```python
from build123d import *

# Parameters (mm, degrees)
BOSS_EXTRUDE1_DEPTH = 25.4
CUT_EXTRUDE1_DEPTH  = 9.5
SKETCH5_W           = 25.4
SKETCH5_H           = 42.164
BOSS_EXTRUDE2_DEPTH = 11.43
CUT_EXTRUDE2_REACH  = 53.538
CUT_EXTRUDE3_REACH  = 53.255
CUT_EXTRUDE4_DEPTH  = 20
SKETCH10_W          = 19.05
SKETCH10_H          = 19.05
CUT_EXTRUDE5_DEPTH  = 26.289
CUT_EXTRUDE6_REACH  = 55.322
SKETCH11_W          = 1.5875
SKETCH11_H          = 12.7
SKETCH12_R          = 0.9921875
CUT_EXTRUDE7_DEPTH  = 51.724378715
CUT_EXTRUDE8_REACH  = 52.836
SKETCH13_R          = 0.9921875
CUT_EXTRUDE9_START  = -7.875
CUT_EXTRUDE9_DEPTH  = 1.225
CUT_EXTRUDE10_START = 7.875
CUT_EXTRUDE10_DEPTH = 1.225
CUT_EXTRUDE11_REACH = 52.836
SKETCH15_W          = 2.45
SKETCH15_H          = 6.35


with BuildPart() as part:
    # Sketch2 → Boss-Extrude1 (new body)
    with BuildSketch(Plane.XY):
        Polygon((12.7, -6.35), (14.2875, -6.35), (14.2875, 6.35), (-14.2875, 6.35), (-14.2875, -6.35), (-12.7, -6.35), (-12.7, -35.814), (12.7, -35.814), align=None)
    extrude(amount=BOSS_EXTRUDE1_DEPTH)

    # Sketch3 → Cut-Extrude1 (cut)
    with BuildSketch(Plane.XY.offset(25.4)):
        with BuildLine():
            Line((2.003122562, 2.3), (2.003122562, -2.3))
            ThreePointArc((2.003122562, -2.3), (-3.05, 0), (2.003122562, 2.3))
        make_face()
    extrude(amount=-CUT_EXTRUDE1_DEPTH, mode=Mode.SUBTRACT)

    # Sketch5 → Boss-Extrude2 (add)
    with BuildSketch(Plane(origin=(0, 0, 0), x_dir=(-1, 0, 0), z_dir=(0, 0, -1))):
        with Locations((0, -14.732)):
            Rectangle(SKETCH5_W, SKETCH5_H)
    extrude(amount=BOSS_EXTRUDE2_DEPTH)

    # Sketch6 → Cut-Extrude2 (cut, up to next)
    with BuildSketch(Plane(origin=(12.7, 0, 0), x_dir=(0, 0, -1), z_dir=(1, 0, 0)), mode=Mode.PRIVATE) as cut_extrude2_sk1:
        Polygon((3.175, -35.814), (11.43, -23.01875), (11.43, -35.814), align=None)
    cut_extrude2_tool1 = extrude(cut_extrude2_sk1.sketch, amount=-CUT_EXTRUDE2_REACH, mode=Mode.PRIVATE) & part.part
    add(cut_extrude2_tool1.solids().sort_by_distance((12.7, -31.548917, -8.678333))[0], mode=Mode.SUBTRACT)

    # Sketch7 → Cut-Extrude3 (cut, up to next)
    with BuildSketch(Plane.XZ.offset(35.814), mode=Mode.PRIVATE) as cut_extrude3_sk1:
        Polygon((-12.7, -11.43), (-12.7, -3.175), (-6.35, -11.43), align=None)
    cut_extrude3_tool1 = extrude(cut_extrude3_sk1.sketch, amount=-CUT_EXTRUDE3_REACH, mode=Mode.PRIVATE) & part.part
    # Sketch7 → Cut-Extrude3 (cut, up to next)
    with BuildSketch(Plane.XZ.offset(35.814), mode=Mode.PRIVATE) as cut_extrude3_sk2:
        Polygon((6.35, -11.43), (12.7, -3.175), (12.7, -11.43), align=None)
    cut_extrude3_tool2 = extrude(cut_extrude3_sk2.sketch, amount=-CUT_EXTRUDE3_REACH, mode=Mode.PRIVATE) & part.part
    add(cut_extrude3_tool1.solids().sort_by_distance((-10.583333, -35.814, -8.678333))[0], mode=Mode.SUBTRACT)
    add(cut_extrude3_tool2.solids().sort_by_distance((10.583333, -35.814, -8.678333))[0], mode=Mode.SUBTRACT)

    # Sketch8 → Cut-Extrude4 (cut)
    with BuildSketch(Plane(origin=(0, 0, -11.43), x_dir=(-1, 0, 0), z_dir=(0, 0, -1))):
        with BuildLine():
            Line((-1.651, 2.859615883), (1.651, 2.859615883))
            ThreePointArc((1.651, 2.859615883), (0, -3.302), (-1.651, 2.859615883))
        make_face()
    extrude(amount=-CUT_EXTRUDE4_DEPTH, mode=Mode.SUBTRACT)

    # Sketch10 → Cut-Extrude5 (cut)
    with BuildSketch(Plane.XZ.offset(35.814)):
        with Locations((0, 12.7)):
            Rectangle(SKETCH10_W, SKETCH10_H)
    extrude(amount=-CUT_EXTRUDE5_DEPTH, mode=Mode.SUBTRACT)

    # Sketch11 → Cut-Extrude6 (cut, up to next)
    with BuildSketch(Plane.XY.offset(25.4), mode=Mode.PRIVATE) as cut_extrude6_sk1:
        with Locations((-13.49375, 0)):
            Rectangle(SKETCH11_W, SKETCH11_H)
    cut_extrude6_tool1 = extrude(cut_extrude6_sk1.sketch, amount=-CUT_EXTRUDE6_REACH, mode=Mode.PRIVATE) & part.part
    # Sketch11 → Cut-Extrude6 (cut, up to next)
    with BuildSketch(Plane.XY.offset(25.4), mode=Mode.PRIVATE) as cut_extrude6_sk2:
        with Locations((13.49375, 0)):
            Rectangle(SKETCH11_W, SKETCH11_H)
    cut_extrude6_tool2 = extrude(cut_extrude6_sk2.sketch, amount=-CUT_EXTRUDE6_REACH, mode=Mode.PRIVATE) & part.part
    add(cut_extrude6_tool1.solids().sort_by_distance((-13.49375, 0, 25.4))[0], mode=Mode.SUBTRACT)
    add(cut_extrude6_tool2.solids().sort_by_distance((13.49375, 0, 25.4))[0], mode=Mode.SUBTRACT)

    # Sketch12 → Cut-Extrude7 (cut, through all)
    with BuildSketch(Plane(origin=(12.7, 0, 0), x_dir=(0, 0, -1), z_dir=(1, 0, 0))):
        with Locations(Location((-20.65, 0, 0), (0, 0, 90))):
            Circle(SKETCH12_R)
    extrude(amount=-CUT_EXTRUDE7_DEPTH, mode=Mode.SUBTRACT)

    # Sketch13 → Cut-Extrude8 (cut, up to next)
    with BuildSketch(Plane(origin=(0, 6.35, 0), x_dir=(1, 0, 0), z_dir=(0, 1, 0)), mode=Mode.PRIVATE) as cut_extrude8_sk1:
        with Locations(Location((0, 1.43, 0), (0, 0, 180))):
            Circle(SKETCH13_R)
    cut_extrude8_tool1 = extrude(cut_extrude8_sk1.sketch, amount=-CUT_EXTRUDE8_REACH, mode=Mode.PRIVATE) & part.part
    add(cut_extrude8_tool1.solids().sort_by_distance((0, 6.35, -1.43))[0], mode=Mode.SUBTRACT)

    # Sketch14 → Cut-Extrude9 (cut, symmetric)
    with BuildSketch(Plane(origin=(0, 0, 0), x_dir=(0, 0, -1), z_dir=(1, 0, 0)).offset(CUT_EXTRUDE9_START)):
        Polygon((-17.475, 1.833087105), (-20.65, 3.666174209), (-23.825, 1.833087105), (-23.825, -1.833087105), (-20.65, -3.666174209), (-17.475, -1.833087105), align=None)
    extrude(amount=CUT_EXTRUDE9_DEPTH, both=True, mode=Mode.SUBTRACT)

    # Sketch14<2> → Cut-Extrude10 (cut, symmetric)
    with BuildSketch(Plane(origin=(0, 0, 0), x_dir=(0, 0, -1), z_dir=(1, 0, 0)).offset(CUT_EXTRUDE10_START)):
        Polygon((-17.475, 1.833087105), (-20.65, 3.666174209), (-23.825, 1.833087105), (-23.825, -1.833087105), (-20.65, -3.666174209), (-17.475, -1.833087105), align=None)
    extrude(amount=CUT_EXTRUDE10_DEPTH, both=True, mode=Mode.SUBTRACT)

    # Sketch15 → Cut-Extrude11 (cut, up to next)
    with BuildSketch(Plane(origin=(0, 6.35, 0), x_dir=(1, 0, 0), z_dir=(0, 1, 0)), mode=Mode.PRIVATE) as cut_extrude11_sk1:
        with Locations((-7.875, -20.65)):
            Rectangle(SKETCH15_W, SKETCH15_H)
    cut_extrude11_tool1 = extrude(cut_extrude11_sk1.sketch, amount=-CUT_EXTRUDE11_REACH, mode=Mode.PRIVATE) & part.part
    # Sketch15 → Cut-Extrude11 (cut, up to next)
    with BuildSketch(Plane(origin=(0, 6.35, 0), x_dir=(1, 0, 0), z_dir=(0, 1, 0)), mode=Mode.PRIVATE) as cut_extrude11_sk2:
        with Locations((7.875, -20.65)):
            Rectangle(SKETCH15_W, SKETCH15_H)
    cut_extrude11_tool2 = extrude(cut_extrude11_sk2.sketch, amount=-CUT_EXTRUDE11_REACH, mode=Mode.PRIVATE) & part.part
    add(cut_extrude11_tool1.solids().sort_by_distance((-7.875, 6.35, 20.65))[0], mode=Mode.SUBTRACT)
    add(cut_extrude11_tool2.solids().sort_by_distance((7.875, 6.35, 20.65))[0], mode=Mode.SUBTRACT)


solid = part.part
```
Part model, mm, in its own coordinate system. A direction names the side the tool comes from. Coordinates: 2 decimals unless noted, no trailing zeros. Loops run counter-clockwise (first coordinate to the right, second up) from the corner with the lowest first, then second, coordinate; pieces in that order, holes last. Notation, with made-up numbers: (70, -15) - (97, -15) arc R16 ccw to (97, 3) - close; hole circle Ø2 at (62.5, 84). An arc over 180 degrees is marked (long way). Write item = value, one per line. Start each with the question number.
Item 1: Cut at B-B, the plane y = -19.5. Give the cut face in (x, z) (3 decimals), and give its area (3 significant figures).
Item 2: 3-axis set-ups, long thin cutter, end or side, ignore diameter. For faces 4 (the cylindrical face through (-0.1, -3.3, -1.6)), 5 (the flat face through (0, -23, 3.175)), 6 (the cylindrical face through (0.129, 4.629, -0.446)), 7 (the cylindrical face through (-2.616, -1.569, 20.716)): which of +Z, -Z, +X, -X, +Y, -Y reach the whole face in a straight line?
Item 3: Mould opens along Y. For faces 1 (the flat face through (0, 0, 15.9)), 2 (the flat face through (7.89, -2.76, 19.08)), 3 (the flat face through (-12.7, -15, 11)) say: released by +Y, released by -Y, zero draft, split by the parting line, or undercut.
Item 4: Cut at D-D, the plane z = 12. Give the cut face in (x, y) (3 decimals).
Item 5: Cut at A-A, the plane x = 0. Give the cut face in (y, z) (3 decimals).
Item 6: Cut at C-C, the plane z = 7. Give the cut face in (x, y) (3 decimals), and give its area (3 significant figures).
Item 7: Flat gauge pins, fed straight in: pin 1 Ø5 at (x, z) = (2.5, 17.5) entering from -Y (3 decimals); pin 2 Ø0.7 at (x, y) = (8, 3) entering from -Z; pin 3 Ø1.2 at (y, z) = (0, 20.65) entering from -X; pin 4 Ø2 at (x, y) = (7.5, -21.5) entering from -Z (3 decimals). Where does each tip first touch, or does it go through?
Item 8: Wall check: L1, parallel to X at y = -31, z = 4 (3 decimals); L2, parallel to Z at x = -3.5, y = -21 (3 decimals); L3, parallel to X at y = 0, z = 19. Give the ranges that are in metal, low to high. Write a range as from..to.
The answers:
q1.outline = (-12.7, -3.175) - (-6.35, -11.43) - (6.35, -11.43) - (12.7, -3.175) - (12.7, 25.4) - (-12.7, 25.4) - close; hole (-9.525, 3.175) - (9.525, 3.175) - (9.525, 22.225) - (-9.525, 22.225) - close
q1.area = 520 mm2
q2.face_4 = -Z
q2.face_5 = -Y
q2.face_6 = +Y
q2.face_7 = +Z
q3.face_1 = undercut
q3.face_2 = released by +Y
q3.face_3 = zero draft
q4.outline = (-12.7, -35.814) - (-9.525, -35.814) - (-9.525, -9.525) - (9.525, -9.525) - (9.525, -35.814) - (12.7, -35.814) - (12.7, 6.35) - (-12.7, 6.35) - close
q5.outline = (-35.814, -3.175) - (-23.019, -11.43) - (-3.302, -11.43) - (-3.302, 8.57) - (2.86, 8.57) - (2.86, -0.438) - (6.35, -0.438) - (6.35, 25.4) - (3.05, 25.4) - (3.05, 15.9) - (-3.05, 15.9) - (-3.05, 25.4) - (-35.814, 25.4) - (-35.814, 22.225) - (-9.525, 22.225) - (-9.525, 3.175) - (-35.814, 3.175) - close; (2.86, -11.43) - (6.35, -11.43) - (6.35, -2.422) - (2.86, -2.422) - close
q6.outline = (-12.7, -35.814) - (-9.525, -35.814) - (-9.525, -9.525) - (9.525, -9.525) - (9.525, -35.814) - (12.7, -35.814) - (12.7, 6.35) - (-12.7, 6.35) - close; hole (-1.651, 2.86) arc R3.302 ccw (long way) to (1.651, 2.86) - close
q6.area = 537 mm2
q7.pin_1 = -9.525
q7.pin_2 = -9.74
q7.pin_3 = through
q7.pin_4 = -11.235
q8.L1 = -12.7..-9.525, 9.525..12.7
q8.L2 = -11.43..3.175, 22.225..25.4
q8.L3 = -12.7..-9.1, -6.65..-3.05, 2..6.65, 9.1..12.7
